```python
from build123d import *

# Parameters (mm, degrees)
F0_W     = 140
F0_H     = 45
F0_R     = 14.2875
F1_DEPTH = 6.4
F3_D     = 8.8
F5_D     = 5.5
F5_DEPTH = 13.5
F5_TIP   = 1.6523667023


with BuildPart() as f1:
    # F0 (on Top) → F1 (new body)
    with BuildSketch(Plane.XY):
        Rectangle(F0_W, F0_H)
        with Locations((47.5, 0)):
            Circle(F0_R, mode=Mode.SUBTRACT)
    extrude(amount=F1_DEPTH)

    # F3 (through all)
    with Locations(Plane(origin=(0, 0, 0), x_dir=(1, 0, 0), z_dir=(0, 0, -1))):
        with Locations((-47.5, 0), (-2.5, 0)):
            Hole(F3_D / 2)

    # F5
    with Locations(Plane(origin=(0, 0, 0), x_dir=(1, 0, 0), z_dir=(0, 0, -1))):
        with Locations((-2.5, -15), (17.5, -15), (17.5, 15), (-2.5, 15)):
            Hole(F5_D / 2, depth=F5_DEPTH)
            with Locations((0, 0, -(F5_DEPTH + F5_TIP / 2))):  # 118° drill point
                Cone(0, F5_D / 2, F5_TIP, mode=Mode.SUBTRACT)


solid = f1.part
```
Can you work these out from the model? Positions are in its coordinate system, mm. Coordinates: 2 decimals unless noted, no trailing zeros. Loops run counter-clockwise (first coordinate to the right, second up) from the corner with the lowest first, then second, coordinate; pieces in that order, holes last. Notation, with made-up numbers: (3, 81.25) -> (36, 81.25) arc R24 cw to (36, 92.25) -> close; hole circle Ø5 at (71.5, -8). An arc over 180 degrees is marked (long way). Answer as a JSON object with one key per item and string values.
1) Imagine slicing it at B-B (z = 1.25). Count the separate pieces of the cut face and the enclosed holes in it, then the cut area to 3 significant figures.
Results:
{"separate pieces": "1", "enclosed holes": "7", "area": "5,440 mm^2"}
2) If I drill on line 1 (Y direction, x = -2.5, z = 2.75); line 2 (X direction, y = 15, z = 4.5); line 3 (Y direction, x = 47.5, z = 3.25), over which ranges is the centre line in solid material (lowest first)?
Results:
{"line 1": "y = -22.5 to -17.75, -12.25 to -4.4, 4.4 to 12.25, 17.75 to 22.5", "line 2": "x = -70 to -5.25, 0.25 to 14.75, 20.25 to 70", "line 3": "y = -22.5 to -14.29, 14.29 to 22.5"}
3) Thinking about a two-plate mould opening in Y: for faces 1 (the face through (-1, 22.5, 3)), 2 (the face through (-3.98, 12.68, 3.24)), 3 (the face through (-2.142, -17.727, 3.245)), 4 (the face through (-1, 5, 0)), which applies, pulls with the +Y half, pulls with the -Y half, needs draft (parallel to the pull), parting line crosses it, or undercut?
Results:
{"face 1": "pulls with the +Y half", "face 2": "undercut", "face 3": "undercut", "face 4": "needs draft"}
4) Imagine slicing it at C-C (x = 17.5). Please give me the cut outline in (y, z).
Results:
{"outline": "(-22.5, 0) -> (-17.75, 0) -> (-17.75, 6.4) -> (-22.5, 6.4) -> close; (-12.25, 0) -> (12.25, 0) -> (12.25, 6.4) -> (-12.25, 6.4) -> close; (17.75, 0) -> (22.5, 0) -> (22.5, 6.4) -> (17.75, 6.4) -> close"}
5) For P1, Ø4.5, axis at x = 17.5, y = -15, coming from the +Z side; P2, Ø10, axis at x = -17.5, y = 0, coming from the -Z side, each with a flat end and sliding along its axis, tell me the tip position at first contact or that it passes through.
Results:
{"P1": "passes through", "P2": "stops at z = 0"}
6) Imagine slicing it at A-A (x = -2.5). Please give me the cut outline in (y, z), then the cut area to 3 significant figures.
Results:
{"outline": "(-22.5, 0) -> (-17.75, 0) -> (-17.75, 6.4) -> (-22.5, 6.4) -> close; (-12.25, 0) -> (-4.4, 0) -> (-4.4, 6.4) -> (-12.25, 6.4) -> close; (4.4, 0) -> (12.25, 0) -> (12.25, 6.4) -> (4.4, 6.4) -> close; (17.75, 0) -> (22.5, 0) -> (22.5, 6.4) -> (17.75, 6.4) -> close", "area": "161 mm^2"}
7) Imagine slicing it at D-D (y = 6). Please give me the cut outline in (x, z).
Results:
{"outline": "(-70, 0) -> (34.53, 0) -> (34.53, 6.4) -> (-70, 6.4) -> close; (60.47, 0) -> (70, 0) -> (70, 6.4) -> (60.47, 6.4) -> close"}
